Geometry: final body of the model. Coordinates: model frame, mm. Face numbers are marked on the shaded views. Coordinates: 2 decimals unless noted, no trailing zeros. Order: outer loops, then holes, each group sorted by start corner. A loop starts at its lowest first (then second) coordinate and runs counter-clockwise, first axis right, second up. Notation, with made-up numbers: (17.25, 32) -> (25.25, 32) arc R17 cw to (25.25, 44) -> close; hole circle Ø5 at (17.25, 49). An arc over 180 degrees is marked (long way). Use one line per item in the form item = value.
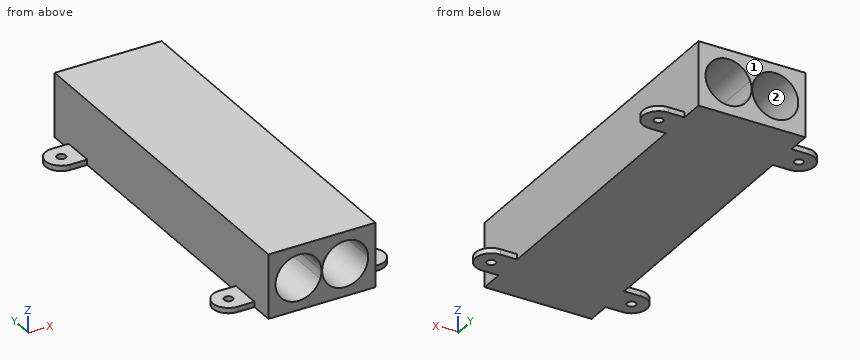
```python
from build123d import *

# Parameters (mm, degrees)
F0_R     = 1.778
F1_DEPTH = 2.159
F2_W     = 43.18
F2_H     = 146.05
F3_DEPTH = 21.59
F4_W     = 43.18
F4_H     = 146.05
F5_DEPTH = 2.159
F7_DEPTH = 146.051


with BuildPart() as f1:
    # F0 (on Top) → F1 (new body)
    with BuildSketch(Plane.XY):
        Polygon((21.59, 63.5), (21.59, 73.025), (-21.59, 73.025), (-21.59, 63.5), (-21.59, 50.8), (-21.59, -50.8), (-21.59, -63.5), (-21.59, -73.025), (21.59, -73.025), (21.59, -63.5), (21.59, -50.8), (21.59, 50.8), align=None)
        with BuildLine():
            Line((28.321, 63.5), (21.59, 63.5))
            Line((21.59, 63.5), (21.59, 50.8))
            Line((21.59, 50.8), (28.321, 50.8))
            ThreePointArc((28.321, 50.8), (34.671, 57.15), (28.321, 63.5))
        make_face()
        with Locations((28.321, 57.15)):
            Circle(F0_R, mode=Mode.SUBTRACT)
        with BuildLine():
            Line((-21.59, 50.8), (-21.59, 63.5))
            Line((-21.59, 63.5), (-28.321, 63.5))
            ThreePointArc((-28.321, 63.5), (-34.671, 57.15), (-28.321, 50.8))
            Line((-28.321, 50.8), (-21.59, 50.8))
        make_face()
        with Locations((-28.321, 57.15)):
            Circle(F0_R, mode=Mode.SUBTRACT)
        with BuildLine():
            Line((28.321, -50.8), (21.59, -50.8))
            Line((21.59, -50.8), (21.59, -63.5))
            Line((21.59, -63.5), (28.321, -63.5))
            ThreePointArc((28.321, -63.5), (34.671, -57.15), (28.321, -50.8))
        make_face()
        with Locations((28.321, -57.15)):
            Circle(F0_R, mode=Mode.SUBTRACT)
        with BuildLine():
            Line((-21.59, -63.5), (-21.59, -50.8))
            Line((-21.59, -50.8), (-28.321, -50.8))
            ThreePointArc((-28.321, -50.8), (-34.671, -57.15), (-28.321, -63.5))
            Line((-28.321, -63.5), (-21.59, -63.5))
        make_face()
        with Locations((-28.321, -57.15)):
            Circle(F0_R, mode=Mode.SUBTRACT)
    extrude(amount=F1_DEPTH)

    # F2 (on face) → F3 (join)
    with BuildSketch(Plane.XY.offset(2.159)):
        Rectangle(F2_W, F2_H)
    extrude(amount=F3_DEPTH)

    # F4 (on face) → F5 (join)
    with BuildSketch(Plane.XY.offset(23.749)):
        Rectangle(F4_W, F4_H)
    extrude(amount=F5_DEPTH)

    # F6 (on face) → F7 (cut, through all)
    with BuildSketch(Plane.XZ.offset(73.025)):
        with BuildLine():
            Line((-0.635, 9.922981), (-0.635, 15.985019))
            ThreePointArc((-0.635, 15.985019), (-18.7198, 12.954), (-0.635, 9.922981))
        make_face()
        with BuildLine():
            ThreePointArc((-0.635, 9.922981), (-0.25488, 11.417352), (-0.127, 12.954))
            ThreePointArc((-0.127, 12.954), (-0.25488, 14.490648), (-0.635, 15.985019))
            Line((-0.635, 15.985019), (-0.635, 9.922981))
        make_face()
        with BuildLine():
            Line((0.635, 9.922981), (0.635, 15.985019))
            ThreePointArc((0.635, 15.985019), (0.127, 12.954), (0.635, 9.922981))
        make_face()
        with BuildLine():
            ThreePointArc((18.7198, 12.954), (10.960048, 22.12252), (0.635, 15.985019))
            Line((0.635, 15.985019), (0.635, 9.922981))
            ThreePointArc((0.635, 9.922981), (10.960048, 3.78548), (18.7198, 12.954))
        make_face()
    extrude(amount=-F7_DEPTH, mode=Mode.SUBTRACT)


solid = f1.part
```
1) Section C-C, the plane z = 19.5. Output: boundary loops of the cut face in (x, y) (3 decimals).
Results found:
outline = (-21.59, -73.025) -> (-16.024, -73.025) -> (-16.024, 73.025) -> (-21.59, 73.025) -> close; (-2.822, -73.025) -> (2.822, -73.025) -> (2.822, 73.025) -> (-2.822, 73.025) -> close; (16.024, -73.025) -> (21.59, -73.025) -> (21.59, 73.025) -> (16.024, 73.025) -> close
2) Section D-D, the plane x = -4. Output: boundary loops of the cut face in (y, z) (3 decimals), and give its area (3 significant figures).
Results found:
outline = (-73.025, 0) -> (73.025, 0) -> (73.025, 5.404) -> (-73.025, 5.404) -> close; (-73.025, 20.504) -> (73.025, 20.504) -> (73.025, 25.908) -> (-73.025, 25.908) -> close
area = 1,580 mm2
3) Section A-A, the plane y = 57.15. Output: boundary loops of the cut face in (x, z) (3 decimals), and give its area (3 significant figures).
Results found:
outline = (-34.671, 0) -> (-30.099, 0) -> (-30.099, 2.159) -> (-34.671, 2.159) -> close; (-26.543, 0) -> (26.543, 0) -> (26.543, 2.159) -> (21.59, 2.159) -> (21.59, 25.908) -> (-21.59, 25.908) -> (-21.59, 2.159) -> (-26.543, 2.159) -> close; (30.099, 0) -> (34.671, 0) -> (34.671, 2.159) -> (30.099, 2.159) -> close; hole (-0.635, 9.923) arc R9.296 ccw to (-0.127, 12.954) arc R9.296 ccw to (-0.635, 15.985) arc R9.296 ccw (long way) to start; hole (0.635, 9.923) arc R9.296 ccw (long way) to (0.635, 15.985) arc R9.296 ccw to start
area = 617 mm2
4) Contact query for flat-ended pins moving along their axis: P1, Ø10, axis at x = 6.5, y = -2, coming from the -Z side; P2, Ø1.7, axis at x = 25, z = 1, coming from the +Y side; P3, Ø2, axis at x = 24.5, z = 5.5, coming from the +Y side; P4, Ø6.5, axis at x = 27, y = -58, coming from the +Z side. Output: stop coordinate, or through.
Results found:
P1 = 0
P2 = 63.5
P3 = through
P4 = 2.16
5) Material intervals for probe 1 along X at (y, z) = (-27, 10.5); probe 2 along X at (y, z) = (45, 18.5); probe 3 along Z at (x, y) = (-10, 31.5), sorted ascending. Write a range as from..to.
Results found:
probe_1 = -21.59..-18.39, -0.46..0.46, 18.39..21.59
probe_2 = -21.59..-16.88, -1.96..1.96, 16.88..21.59
probe_3 = 0..3.68, 22.23..25.91
6) Pull-direction query (X, two-part tool) for the marked faces 1 and 2; classes: released by +X, released by -X, zero draft, split by the parting line, or undercut.
Results found:
face_1 = zero draft
face_2 = undercut
7) Section B-B, the plane x = -25. Output: boundary loops of the cut face in (y, z), and give its area (3 significant figures).
Results found:
outline = (-63.5, 0) -> (-50.8, 0) -> (-50.8, 2.16) -> (-63.5, 2.16) -> close; (50.8, 0) -> (63.5, 0) -> (63.5, 2.16) -> (50.8, 2.16) -> close
area = 54.8 mm2
